```python
from build123d import *

# Parameters (mm, degrees)
SKETCH1_R               = 3
SKETCH1_R_2             = 7.95
MAIN_BODY_LINK_B1_DEPTH = 6
CUT_EXTRUDE1_REACH      = 169.025
CUT_EXTRUDE2_REACH      = 169.025
SKETCH3_R               = 1.5
FILLET1_R               = 1
SKETCH4_R               = 15.25
CUT_EXTRUDE3_DEPTH      = 168.02546447


with BuildPart() as part:
    # Sketch1 → Main Body Link B1 (new body)
    with BuildSketch(Plane.XY):
        with BuildLine():
            Line((-11.1, 83.474052381), (-9.1, 83.474052381))
            Line((-9.1, 83.474052381), (0, 83.474052381))
            Line((0, 83.474052381), (9.1, 83.474052381))
            Line((9.1, 83.474052381), (11.1, 83.474052381))
            Line((11.1, 83.474052381), (20.2, 83.474052381))
            Line((20.2, 83.474052381), (20.2, 90.874052381))
            Line((20.2, 90.874052381), (17.986683974, 148.383116621))
            ThreePointArc((17.986683974, 148.383116621), (0, 165.690874165), (-17.986683974, 148.383116621))
            Line((-17.986683974, 148.383116621), (-20.2, 90.874052381))
            Line((-20.2, 90.874052381), (-20.2, 83.474052381))
            Line((-20.2, 83.474052381), (-11.1, 83.474052381))
        make_face()
        with Locations((5.2, 88.124052381)):
            Circle(SKETCH1_R, mode=Mode.SUBTRACT)
        with Locations((15, 88.124052381)):
            Circle(SKETCH1_R, mode=Mode.SUBTRACT)
        with Locations((-15, 88.124052381)):
            Circle(SKETCH1_R, mode=Mode.SUBTRACT)
        with Locations((-5.2, 88.124052381)):
            Circle(SKETCH1_R, mode=Mode.SUBTRACT)
        with Locations((0, 147.690874165)):
            Circle(SKETCH1_R_2, mode=Mode.SUBTRACT)
    extrude(amount=MAIN_BODY_LINK_B1_DEPTH)

    # Sketch2 → Cut-Extrude1 (cut, up to next)
    with BuildSketch(Plane.XY.offset(6), mode=Mode.PRIVATE) as cut_extrude1_sk1:
        Polygon((-3.278172542, 117.482670232), (12, 128.172168466), (12, 106.793171999), align=None)
    cut_extrude1_tool1 = extrude(cut_extrude1_sk1.sketch, amount=-CUT_EXTRUDE1_REACH, mode=Mode.PRIVATE) & part.part
    # Sketch2 → Cut-Extrude1 (cut, up to next)
    with BuildSketch(Plane.XY.offset(6), mode=Mode.PRIVATE) as cut_extrude1_sk2:
        with BuildLine():
            ThreePointArc((-12, 134.2744663), (-7.774454217, 131.456408925), (-2.929911079, 129.930929878))
            Line((-2.929911079, 129.930929878), (-12, 123.584968066))
            Line((-12, 123.584968066), (-12, 134.2744663))
        make_face()
    cut_extrude1_tool2 = extrude(cut_extrude1_sk2.sketch, amount=-CUT_EXTRUDE1_REACH, mode=Mode.PRIVATE) & part.part
    # Sketch2 → Cut-Extrude1 (cut, up to next)
    with BuildSketch(Plane.XY.offset(6), mode=Mode.PRIVATE) as cut_extrude1_sk3:
        Polygon((-12, 111.380372399), (-12, 100.690874165), (3.278172542, 100.690874165), align=None)
    cut_extrude1_tool3 = extrude(cut_extrude1_sk3.sketch, amount=-CUT_EXTRUDE1_REACH, mode=Mode.PRIVATE) & part.part
    add(cut_extrude1_tool1.solids().sort_by_distance((6.907276, 117.48267, 6))[0], mode=Mode.SUBTRACT)
    add(cut_extrude1_tool2.solids().sort_by_distance((-9.12997, 128.978342, 6))[0], mode=Mode.SUBTRACT)
    add(cut_extrude1_tool3.solids().sort_by_distance((-6.907276, 104.25404, 6))[0], mode=Mode.SUBTRACT)

    # Sketch3 → Cut-Extrude2 (cut, up to next)
    with BuildSketch(Plane.XY.offset(6), mode=Mode.PRIVATE) as cut_extrude2_sk1:
        with Locations((-11.5, 147.690874165)):
            Circle(SKETCH3_R)
    cut_extrude2_tool1 = extrude(cut_extrude2_sk1.sketch, amount=-CUT_EXTRUDE2_REACH, mode=Mode.PRIVATE) & part.part
    # Sketch3 → Cut-Extrude2 (cut, up to next)
    with BuildSketch(Plane.XY.offset(6), mode=Mode.PRIVATE) as cut_extrude2_sk2:
        with Locations((11.5, 147.690874165)):
            Circle(SKETCH3_R)
    cut_extrude2_tool2 = extrude(cut_extrude2_sk2.sketch, amount=-CUT_EXTRUDE2_REACH, mode=Mode.PRIVATE) & part.part
    add(cut_extrude2_tool1.solids().sort_by_distance((-11.5, 147.690874, 6))[0], mode=Mode.SUBTRACT)
    add(cut_extrude2_tool2.solids().sort_by_distance((11.5, 147.690874, 6))[0], mode=Mode.SUBTRACT)

    # Fillet1
    fillet1_edges = [part.edges().sort_by_distance(p)[0] for p in [
        (-3.278172542, 117.482670232, 3),
        (12, 128.172168466, 3),
        (12, 106.793171999, 3),
        (-12, 134.2744663, 3),
        (-2.929911079, 129.930929878, 3),
        (-12, 123.584968066, 3),
        (-12, 111.380372399, 3),
        (3.278172542, 100.690874165, 3),
        (-12, 100.690874165, 3),
    ]]
    fillet(fillet1_edges, radius=FILLET1_R)

    # Sketch4 → Cut-Extrude3 (cut, through all)
    with BuildSketch(Plane.XY.offset(6)):
        with Locations((0, 147.690874165)):
            Circle(SKETCH4_R)
    extrude(amount=-CUT_EXTRUDE3_DEPTH, mode=Mode.SUBTRACT)


solid = part.part
```
Design review of the part built by this model. Coordinates are the model's own, in mm. A direction names the side the tool comes from. Round coordinates to 2 decimals unless told otherwise and drop trailing zeros. Write each loop counter-clockwise with the first axis right and the second up, starting at its lowest first coordinate (ties: lowest second). Pieces come first, ordered by that corner, then holes. Notation, with made-up numbers: (50.5, -36.5) -> (69.5, -36.5) arc R27 ccw to (69.5, -7.5) -> close; hole circle Ø8 at (-40, 81.5). An arc over 180 degrees is marked (long way). Write item = value, one per line. Start each with the question number.
1) Clearance check with flat-ended pins moving along their axes: pin 1 (3 mm diameter, centred on x = -7, z = 3.5, fed in from +Y); pin 2 (1.5 mm diameter, centred on y = 112, z = 2.5, fed in from -X); pin 3 (1.8 mm diameter, centred on y = 104.5, z = 3, fed in from +X). State where each tip first meets the part, or that it passes through.
2) Take a section at B-B, the plane y = 105.5. State the section outline as (x, z) points, plus the area to 3 significant figures.
3) Mouldability with a two-part tool opening along Y and no side actions: class faces 3 (the face through (12, 118, 3)), 4 (the face through (0, 83.474, 3)), 5 (the face through (-12.1, 138.41, 3.04)), 6 (the face through (19.11, 119.23, 2.96)) as +Y half, -Y half, draft (parallel to the pull), parting line (faces both ways), or undercut.
4) Take a section at C-C, the plane x = -16.5. State the section outline as (y, z) points, plus the area to 3 significant figures.
5) Tool access review of faces 1 (the face through (20.2, 87, 3)), 2 (the face through (-6, 100.691, 3)): name each direction out of +Z, -Z, +X, -X, +Y, -Y from which nothing blocks a thin tool from reaching the whole face with its end or side.
6) Take a section at D-D, the plane z = 4.75. Count the separate pieces of the cut face and the enclosed holes in it, plus the area to 3 significant figures.
7) Take a section at A-A, the plane x = 5.2. State the section outline as (y, z) points, plus the area to 3 significant figures.
8) Wall thickness on probe 1 along X at (y, z) = (90, 4); probe 2 along Y at (x, z) = (-5.2, 3.45); probe 3 along Y at (x, z) = (5.2, 2.9): over which ranges is each line inside the solid? List them lowest first. Write a range as from..to.
Results list:
q1.pin_1 = 164.83
q1.pin_2 = -19.42
q1.pin_3 = 19.71
q2.outline = (-19.64, 0) -> (-12, 0) -> (-12, 6) -> (-19.64, 6) -> close; (-3.6, 0) -> (19.64, 0) -> (19.64, 6) -> (-3.6, 6) -> close
q2.area = 185 mm²
q3.face_3 = undercut
q3.face_4 = -Y half
q3.face_5 = undercut
q3.face_6 = +Y half
q4.outline = (83.47, 0) -> (85.53, 0) -> (85.53, 6) -> (83.47, 6) -> close; (90.72, 0) -> (154.88, 0) -> (154.88, 6) -> (90.72, 6) -> close
q4.area = 397 mm²
q5.face_1 = +Z, -Z, +X, +Y, -Y
q5.face_2 = +Z, -Z
q6.separate_pieces = 1
q6.enclosed_holes = 8
q6.area = 1,850 mm²
q7.outline = (83.47, 0) -> (85.12, 0) -> (85.12, 6) -> (83.47, 6) -> close; (91.12, 0) -> (111.55, 0) -> (111.55, 6) -> (91.12, 6) -> close; (123.41, 0) -> (133.35, 0) -> (133.35, 6) -> (123.41, 6) -> close; (162.03, 0) -> (164.92, 0) -> (164.92, 6) -> (162.03, 6) -> close
q7.area = 209 mm²
q8.probe_1 = -20.2..-17.34, -12.66..-7.54, -2.86..2.86, 7.54..12.66, 17.34..20.2
q8.probe_2 = 83.47..85.12, 91.12..100.69, 106.62..128.34, 130.46..133.35, 162.03..164.92
q8.probe_3 = 83.47..85.12, 91.12..111.55, 123.41..133.35, 162.03..164.92
